Geometry check sheet. Reference: drawing and pictorial views, mm from the part's lowest x, y, z. A direction names the side the tool comes from. Round coordinates to 2 decimals unless told otherwise and drop trailing zeros. Order: outer loops, then holes, each group sorted by start corner. A loop starts at its lowest first (then second) coordinate and runs counter-clockwise, first axis right, second up.
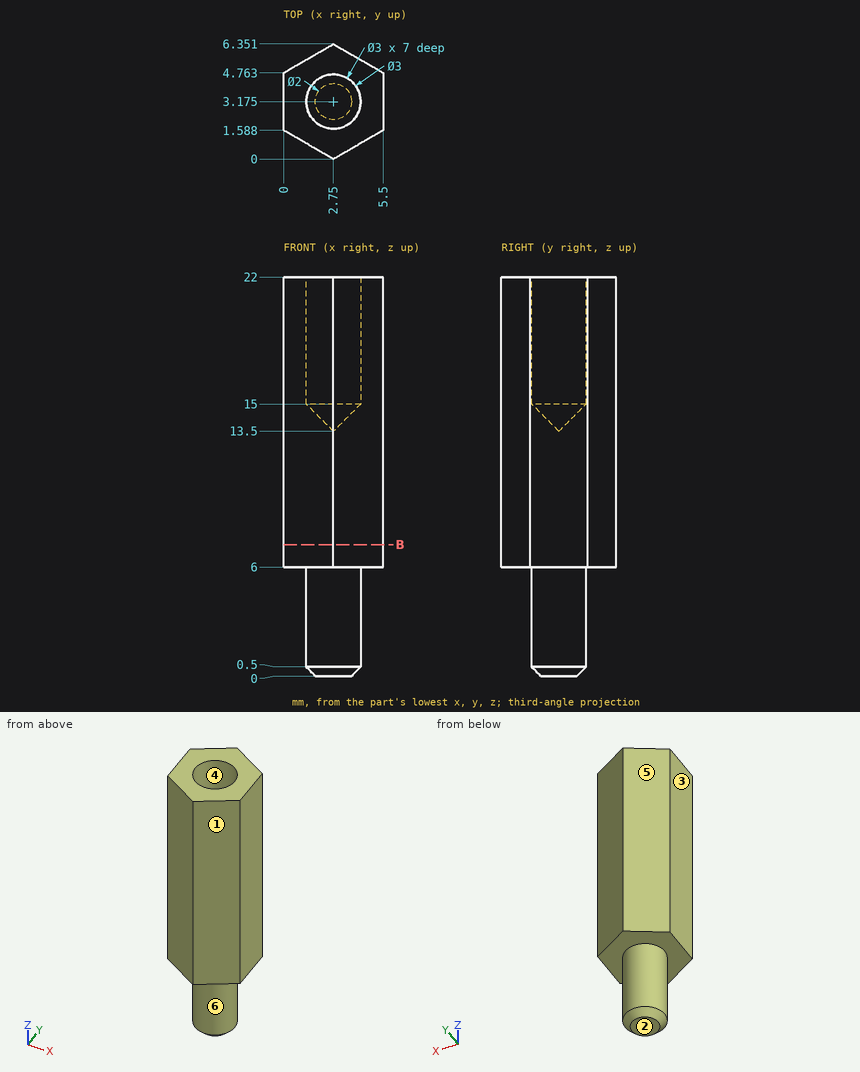
1) Sectioned sample at B-B on z = 7.25. Record the cut outline in (x, y), then the cut area to 3 significant figures.
2) Tool access check on the marked faces 5 and 6. Record the directions out of +Z, -Z, +X, -X, +Y, -Y that give a thin tool (end or side, any length) a straight path to the whole face; none if there is none.
3) Draft check along X on the marked faces 1, 2, 3 and 4. Enter one of: released by +X, released by -X, zero draft, split by the parting line, or undercut.
4) Go/stop test with flat-tipped pins: pin 1 Ø2 at (x, z) = (0.5, 19) entering from -Y; pin 2 Ø2.5 at (x, y) = (2.75, 3.18) entering from +Z (1 decimal); pin 3 Ø1.5 at (x, y) = (1, 4) entering from -Z (1 decimal). Record where each tip stops, or that it passes through.
5) Scan lines: probe 1 along Z at (x, y) = (2.75, 5.5); probe 2 along Y at (x, z) = (1.5, 20.5) (1 decimal); probe 3 along X at (y, z) = (3, 17). Record each from-to range of solid material in increasing order.
Returned:
1. outline: (0, 1.59) - (2.75, 0) - (5.5, 1.59) - (5.5, 4.76) - (2.75, 6.35) - (0, 4.76) - close
1. area: 26.2 mm2
2. face 5: +Z, -Z, -X, +Y
2. face 6: -Z
3. face 1: released by +X
3. face 2: zero draft
3. face 3: released by -X
3. face 4: undercut
4. pin 1: stops at y = 0.72
4. pin 2: stops at z = 14.8
4. pin 3: stops at z = 0.2
5. probe 1: z = 6 to 22
5. probe 2: y = 0.7 to 2.3, 4 to 5.6
5. probe 3: x = 0 to 1.26, 4.24 to 5.5
